from build123d import *

# Parameters (mm, degrees)
SKETCH1_R           = 2
SKETCH1_R_2         = 2.5
BOSS_EXTRUDE1_DEPTH = 6
FILLET1_R           = 2


with BuildPart() as part:
    # Sketch1 → Boss-Extrude1 (new body)
    with BuildSketch(Plane(origin=(0, 0, 0), x_dir=(1, 0, 0), z_dir=(0, 1, 0))):
        Polygon((-9, 14.125), (-9, -5.875), (14, -5.875), (14, -25), (26, -25), (26, 14.125), align=None)
        with Locations((0, 8.25)):
            Circle(SKETCH1_R, mode=Mode.SUBTRACT)
        Circle(SKETCH1_R, mode=Mode.SUBTRACT)
        with Locations((20, -19)):
            Circle(SKETCH1_R_2, mode=Mode.SUBTRACT)
    extrude(amount=BOSS_EXTRUDE1_DEPTH)

    # Fillet1
    fillet1_edges = [part.edges().sort_by_distance(p)[0] for p in [
        (14, 3, 25),
        (14, 3, 5.875),
        (-9, 3, 5.875),
        (-9, 3, -14.125),
        (26, 3, -14.125),
        (26, 3, 25),
    ]]
    fillet(fillet1_edges, radius=FILLET1_R)


solid = part.part
The listing builds one solid part. Answer for the finished solid, in the listing's coordinates (mm). A direction names the side the tool comes from. Round coordinates to 2 decimals unless told otherwise and drop trailing zeros. Order: outer loops, then holes, each group sorted by start corner. A loop starts at its lowest first (then second) coordinate and runs counter-clockwise, first axis right, second up. Notation, with made-up numbers: (80.25, 18) - (121.25, 18) arc R14 ccw to (121.25, 32) - close; hole circle Ø2 at (9, 60). An arc over 180 degrees is marked (long way). Write item = value, one per line. Start each with the question number.
1) For a pull along Z with two mould halves and no side action, classify faces 3 (the cylindrical face through (25.399, 3.042, -13.555)), 4 (the cylindrical face through (17.5, 3, 18.9)), 5 (the flat face through (12, 6, 1)) as released by +Z, released by -Z, zero draft, split by the parting line, or undercut.
2) For faces 1 (the cylindrical face through (-8.43, 3.042, -13.524)), 2 (the flat face through (14, 3, 15)), determine the directions among +Z, -Z, +X, -X, +Y, -Y from which every point of the face is accessible in a straight line to the end or side of a thin tool.
3) Section B-B, the plane z = 19 is taken. Write down the section's boundary in (x, y).
4) Section D-D, the plane y = 2.35 is taken. Write down the section's boundary in (x, z) (3 decimals).
5) Given pin 1 (2 mm diameter, centred on x = 7.5, y = 1.5, fed in from +Z) (3 decimals), flat-ended and moving along its own axis, determine where the tip first touches the part or whether it passes through.
6) Section C-C, the plane x = 18 is taken. Write down the section's boundary in (y, z) (3 decimals), plus the area to 3 significant figures.
7) Section A-A, the plane x = 0 is taken. Write down the section's boundary in (y, z) (3 decimals).
8) Straight lines are drawn through the part: L1, parallel to Z at x = 0, y = 3.75 (3 decimals); L2, parallel to X at y = 4.1, z = 0; L3, parallel to Z at x = 20, y = 2.75 (3 decimals). For each, find the intervals that lie inside material, in ascending order.
Results list:
q1.face_3 = released by -Z
q1.face_4 = undercut
q1.face_5 = zero draft
q2.face_1 = -Z, -X, +Y, -Y
q2.face_2 = +Z, -X, +Y, -Y
q3.outline = (14, 0) - (17.5, 0) - (17.5, 6) - (14, 6) - close; (22.5, 0) - (26, 0) - (26, 6) - (22.5, 6) - close
q4.outline = (-9, -12.125) arc R2 ccw to (-7, -14.125) - (24, -14.125) arc R2 ccw to (26, -12.125) - (26, 23) arc R2 ccw to (24, 25) - (16, 25) arc R2 ccw to (14, 23) - (14, 7.875) arc R2 cw to (12, 5.875) - (-7, 5.875) arc R2 ccw to (-9, 3.875) - close; hole circle Ø4 at (0, -8.25); hole circle Ø4 at (0, 0); hole circle Ø5 at (20, 19)
q5.pin_1 = 5.875
q6.outline = (0, -14.125) - (6, -14.125) - (6, 17.5) - (0, 17.5) - close; (0, 20.5) - (6, 20.5) - (6, 25) - (0, 25) - close
q6.area = 217 mm^2
q7.outline = (0, -14.125) - (6, -14.125) - (6, -10.25) - (0, -10.25) - close; (0, -6.25) - (6, -6.25) - (6, -2) - (0, -2) - close; (0, 2) - (6, 2) - (6, 5.875) - (0, 5.875) - close
q8.L1 = -14.125 to -10.25, -6.25 to -2, 2 to 5.875
q8.L2 = -9 to -2, 2 to 26
q8.L3 = -14.125 to 16.5, 21.5 to 25
